```python
from build123d import *

# Parameters (mm, degrees)
BOSS_EXTRUDE1_DEPTH = 6.35


with BuildPart() as part:
    # Sketch1 → Boss-Extrude1 (new body)
    with BuildSketch(Plane(origin=(0, 0, 0), x_dir=(1, 0, 0), z_dir=(0, 1, 0))):
        Polygon((152.4, 152.4), (6.35, 152.4), (6.35, 127), (0, 127), (0, 101.6), (6.35, 101.6), (6.35, 82.55), (0, 82.55), (0, 44.45), (6.35, 44.45), (6.35, 0), (44.45, 0), (44.45, 6.35), (82.55, 6.35), (82.55, 0), (101.6, 0), (101.6, 6.35), (127, 6.35), (127, 0), (152.4, 0), align=None)
        Polygon((6.35, 177.8), (6.35, 152.4), (152.4, 152.4), (152.4, 304.8), (127, 304.8), (127, 298.45), (101.6, 298.45), (101.6, 304.8), (82.55, 304.8), (82.55, 298.45), (44.45, 298.45), (44.45, 304.8), (6.35, 304.8), (6.35, 260.35), (0, 260.35), (0, 222.25), (6.35, 222.25), (6.35, 203.2), (0, 203.2), (0, 177.8), align=None)
        Polygon((152.4, 304.8), (152.4, 152.4), (298.45, 152.4), (298.45, 177.8), (304.8, 177.8), (304.8, 203.2), (298.45, 203.2), (298.45, 222.25), (304.8, 222.25), (304.8, 260.35), (298.45, 260.35), (298.45, 304.8), (260.35, 304.8), (260.35, 298.45), (222.25, 298.45), (222.25, 304.8), (203.2, 304.8), (203.2, 298.45), (177.8, 298.45), (177.8, 304.8), align=None)
        Polygon((298.45, 152.4), (152.4, 152.4), (152.4, 0), (177.8, 0), (177.8, 6.35), (203.2, 6.35), (203.2, 0), (222.25, 0), (222.25, 6.35), (260.35, 6.35), (260.35, 0), (298.45, 0), (298.45, 44.45), (304.8, 44.45), (304.8, 82.55), (298.45, 82.55), (298.45, 101.6), (304.8, 101.6), (304.8, 127), (298.45, 127), align=None)
    extrude(amount=BOSS_EXTRUDE1_DEPTH)


solid = part.part
```
Can you work these out from the model? Positions are in its coordinate system, mm. Coordinates: 2 decimals unless noted, no trailing zeros. Write each loop counter-clockwise with the first axis right and the second up, starting at its lowest first coordinate (ties: lowest second). Pieces come first, ordered by that corner, then holes. Notation, with made-up numbers: (16, -29) - (27, -29) arc R11 ccw to (27, -8) - close; hole circle Ø2 at (44, 72). An arc over 180 degrees is marked (long way). Return JSON: item names as keys, results as strings.
Q1. If we section it at A-A (x = 196): Please give me the cut outline in (y, z).
Computed values:
{"outline": "(0, -298.45) - (6.35, -298.45) - (6.35, -6.35) - (0, -6.35) - close"}
Q2. Please list where these lines run through material, in increasing order: L1, parallel to Z at x = 231, y = 1.5; L2, parallel to X at y = 3.5, z = -218.5. Write a range as from..to.
Computed values:
{"L1": "z = -298.45..-6.35", "L2": "x = 6.35..298.45"}
Q3. I'm going to push flat-ended pins straight in: pin 1 Ø3 at (x, y) = (4.5, 4) entering from -Z; pin 2 Ø3 at (y, z) = (3, -209) entering from +X; pin 3 Ø1.9 at (x, y) = (185.5, 3) entering from +Z. Where does each tip first touch, or does it pass through?
Computed values:
{"pin 1": "stops at z = -260.35", "pin 2": "stops at x = 298.45", "pin 3": "stops at z = -6.35"}
Q4. If we section it at B-B (z = -158.5): Please give me the cut outline in (x, y), then the cut area to 3 significant figures.
Computed values:
{"outline": "(6.35, 0) - (298.45, 0) - (298.45, 6.35) - (6.35, 6.35) - close", "area": "1,850 mm2"}
